```python
from build123d import *

# Parameters (mm, degrees)
BOSS_EXTRUDE4_DEPTH  = 1.5875
M3_CLEARANCE_HOLE3_D = 3
M3_CLEARANCE_HOLE1_D = 3.1
M3_CLEARANCE_HOLE4_D = 2.95
M3_CLEARANCE_HOLE2_D = 3.1
BOSS_EXTRUDE6_DEPTH  = 3.175
FILLET1_R            = 2
FILLET3_R            = 1
FILLET6_R            = 0.5
SKETCH28_W           = 54.5
SKETCH28_H           = 45
CUT_EXTRUDE4_DEPTH   = 10
CUT_EXTRUDE5_DEPTH   = 10
SKETCH30_W           = 42
SKETCH30_H           = 26
CUT_EXTRUDE6_DEPTH   = 10
SKETCH31_R           = 1.5
CUT_EXTRUDE7_DEPTH   = 10
SKETCH34_R           = 1
CUT_EXTRUDE9_DEPTH   = 10
SKETCH35_R           = 1.5
CUT_EXTRUDE10_DEPTH  = 121.250075508


with BuildPart() as part:
    # Sketch1 → Boss-Extrude4 (new, symmetric)
    with BuildSketch(Plane(origin=(0, 0, 0), x_dir=(1, 0, 0), z_dir=(0, 1, 0))):
        with BuildLine():
            Line((-62.799553621, 32.496136604), (-73.969425011, 32.691107434))
            Line((-73.969425011, 32.691107434), (-77.053684287, 35.88495141))
            ThreePointArc((-77.053684287, 35.88495141), (-84.36642289, 10.358894189), (-83.446216027, -16.178041625))
            Line((-83.446216027, -16.178041625), (-79.680911643, -13.825218315))
            Line((-79.680911643, -13.825218315), (-69.484649137, -16.179210996))
            Line((-69.484649137, -16.179210996), (-43.894490772, -57.132025032))
            Line((-43.894490772, -57.132025032), (-43.894490772, -64.826600275))
            Line((-43.894490772, -64.826600275), (-43.094490772, -64.826600275))
            Line((-43.094490772, -64.826600275), (-34, -64.826600275))
            Line((-34, -64.826600275), (-34, -62.55))
            Line((-34, -62.55), (-34, -61.55))
            Line((-34, -61.55), (-20, -61.55))
            Line((-20, -61.55), (-19.859459165, -62.55))
            Line((-19.859459165, -62.55), (19.859459165, -62.55))
            Line((19.859459165, -62.55), (20, -61.55))
            Line((20, -61.55), (34, -61.55))
            Line((34, -61.55), (34, -62.55))
            Line((34, -62.55), (34, -64.826600275))
            Line((34, -64.826600275), (43.094490772, -64.826600275))
            Line((43.094490772, -64.826600275), (43.894490772, -64.826600275))
            Line((43.894490772, -64.826600275), (43.894490772, -57.132025032))
            Line((43.894490772, -57.132025032), (69.484649137, -16.179210996))
            Line((69.484649137, -16.179210996), (79.680911643, -13.825218315))
            Line((79.680911643, -13.825218315), (83.446216027, -16.178041625))
            ThreePointArc((83.446216027, -16.178041625), (84.610662337, -8.126242604), (85, 0))
            ThreePointArc((85, 0), (82.98964744, 18.377116688), (77.053684287, 35.88495141))
            Line((77.053684287, 35.88495141), (73.969425011, 32.691107434))
            Line((73.969425011, 32.691107434), (62.799553621, 32.496136604))
            Line((62.799553621, 32.496136604), (30.284668021, 63.895396642))
            Line((30.284668021, 63.895396642), (30.089697191, 75.065268032))
            Line((30.089697191, 75.065268032), (33.173956467, 78.259112008))
            ThreePointArc((33.173956467, 78.259112008), (0, 85), (-33.173956467, 78.259112008))
            Line((-33.173956467, 78.259112008), (-30.089697191, 75.065268032))
            Line((-30.089697191, 75.065268032), (-30.284668021, 63.895396642))
            Line((-30.284668021, 63.895396642), (-62.799553621, 32.496136604))
        make_face()
    extrude(amount=BOSS_EXTRUDE4_DEPTH, both=True)

    # M3 Clearance Hole3 (through all)
    with Locations(Plane(origin=(0, -1.5875, 0), x_dir=(-1, 0, 0), z_dir=(0, -1, 0))):
        with Locations((36.5, -50), (36.5, -38), (-36.5, -50), (-36.5, -38)):
            Hole(M3_CLEARANCE_HOLE3_D / 2)

    # M3 Clearance Hole1 (through all)
    with Locations(Plane(origin=(0, 1.5875, 0), x_dir=(1, 0, 0), z_dir=(0, 1, 0))):
        with Locations((-78.542321426, -8.49139241), (78.542321426, -8.49139241), (74.155025063, 27.240269049), (-74.155025063, 27.240269049)):
            Hole(M3_CLEARANCE_HOLE1_D / 2)

    # M3 Clearance Hole4 (through all)
    with Locations(Plane(origin=(0, -1.5875, 0), x_dir=(-1, 0, 0), z_dir=(0, -1, 0))):
        with Locations((-67.099301622, -15.278865202), (-50.141885166, -42.416404279), (-61.062544382, 30.698137949), (-38.043670771, 52.927205804), (50.141885166, -42.416404279), (67.099301622, -15.278865202), (38.043670771, 52.927205804), (61.062544382, 30.698137949)):
            Hole(M3_CLEARANCE_HOLE4_D / 2)

    # M3 Clearance Hole2 (through all)
    with Locations(Plane(origin=(0, 1.5875, 0), x_dir=(1, 0, 0), z_dir=(0, 1, 0))):
        with Locations((27, 76.497766718), (-27, 76.497766718)):
            Hole(M3_CLEARANCE_HOLE2_D / 2)

    # Sketch22 → Boss-Extrude6 (add)
    with BuildSketch(Plane(origin=(0, 1.5875, 0), x_dir=(1, 0, 0), z_dir=(0, 1, 0))):
        Polygon((65.061950694, 32.535626892), (30.245177733, 66.157793715), (30.284668021, 63.895396642), (62.799553621, 32.496136604), align=None)
        Polygon((-30.284668021, 63.895396642), (-30.245177733, 66.157793715), (-65.061950694, 32.535626892), (-62.799553621, 32.496136604), align=None)
        Polygon((43.894490772, -60.151352895), (71.689396914, -15.670204865), (69.484649137, -16.179210996), (43.894490772, -57.132025032), align=None)
        Polygon((-69.484649137, -16.179210996), (-71.689396914, -15.670204865), (-43.894490772, -60.151352895), (-43.894490772, -57.132025032), align=None)
    extrude(amount=-BOSS_EXTRUDE6_DEPTH)

    # Fillet1
    fillet1_edges = [part.edges().sort_by_distance(p)[0] for p in [
        (-30.245177733, 0.79375, -66.157793715),
        (-65.061950694, 0.79375, -32.535626892),
        (-71.689396914, 0.79375, 15.670204865),
        (-43.894490772, 0.79375, 60.151352895),
        (43.894490772, -0.79375, 60.151352895),
        (71.689396914, -0.79375, 15.670204865),
        (65.061950694, 0.79375, -32.535626892),
        (30.245177733, -0.79375, -66.157793715),
        (30.089697191, -0.79375, -75.065268032),
        (73.969425011, -0.79375, -32.691107434),
        (79.680911643, -0.79375, 13.825218315),
        (-79.680911643, -0.79375, 13.825218315),
        (-73.969425011, -0.79375, -32.691107434),
        (-30.089697191, -0.79375, -75.065268032),
    ]]
    fillet(fillet1_edges, radius=FILLET1_R)

    # Fillet3
    fillet3_edges = [part.edges().sort_by_distance(p)[0] for p in [
        (33.173956467, -0.79375, -78.259112008),
        (77.053684287, 0.79375, -35.88495141),
        (83.446216027, -0.79375, 16.178041625),
        (43.894490772, -0.79375, 64.826600275),
        (34, 0.79375, 64.826600275),
        (34, -0.79375, 61.55),
        (-34, -0.79375, 61.55),
        (-34, 0.79375, 64.826600275),
        (-43.894490772, -0.79375, 64.826600275),
        (-83.446216027, -0.79375, 16.178041625),
        (-77.053684287, -0.79375, -35.88495141),
        (-33.173956467, -0.79375, -78.259112008),
    ]]
    fillet(fillet3_edges, radius=FILLET3_R - 0.0001)  # a hair under: the kernel refuses the full size

    # Fillet6
    fillet6_edges = [part.edges().sort_by_distance(p)[0] for p in [
        (20, -0.79375, 61.55),
        (19.859459165, -0.79375, 62.55),
        (-19.859459165, 0.79375, 62.55),
        (-20, 0.79375, 61.55),
    ]]
    fillet(fillet6_edges, radius=FILLET6_R)

    # Sketch28 → Cut-Extrude4 (cut)
    with BuildSketch(Plane(origin=(0, 1.5875, 0), x_dir=(1, 0, 0), z_dir=(0, 1, 0))):
        with Locations((0, -40.05)):
            Rectangle(SKETCH28_W, SKETCH28_H)
    extrude(amount=-CUT_EXTRUDE4_DEPTH, mode=Mode.SUBTRACT)

    # Sketch29 → Cut-Extrude5 (cut)
    with BuildSketch(Plane(origin=(0, 1.5875, 0), x_dir=(1, 0, 0), z_dir=(0, 1, 0))):
        with BuildLine():
            ThreePointArc((-31.5, -56.8), (-30, -58.3), (-28.5, -56.8))
            Line((-28.5, -56.8), (-30, -56.8))
            Line((-30, -56.8), (-31.5, -56.8))
        make_face()
        with BuildLine():
            Line((-30, -56.8), (-28.5, -56.8))
            ThreePointArc((-28.5, -56.8), (-30, -55.3), (-31.5, -56.8))
            Line((-31.5, -56.8), (-30, -56.8))
        make_face()
        with BuildLine():
            ThreePointArc((28.5, -56.8), (30, -58.3), (31.5, -56.8))
            ThreePointArc((31.5, -56.8), (30, -55.3), (28.5, -56.8))
        make_face()
    extrude(amount=-CUT_EXTRUDE5_DEPTH, mode=Mode.SUBTRACT)

    # Sketch30 → Cut-Extrude6 (cut)
    with BuildSketch(Plane(origin=(0, 1.5875, 0), x_dir=(1, 0, 0), z_dir=(0, 1, 0))):
        with Locations((0, -4.55)):
            Rectangle(SKETCH30_W, SKETCH30_H)
    extrude(amount=-CUT_EXTRUDE6_DEPTH, mode=Mode.SUBTRACT)

    # Sketch31 → Cut-Extrude7 (cut)
    with BuildSketch(Plane(origin=(0, 1.5875, 0), x_dir=(1, 0, 0), z_dir=(0, 1, 0))):
        with Locations(Location((-26, -14.8, 0), (0, 0, 270))):
            Circle(SKETCH31_R)
        with Locations(Location((26, -14.8, 0), (0, 0, 270))):
            Circle(SKETCH31_R)
    extrude(amount=-CUT_EXTRUDE7_DEPTH, mode=Mode.SUBTRACT)

    # Sketch34 → Cut-Extrude9 (cut)
    with BuildSketch(Plane(origin=(0, 1.5875, 0), x_dir=(1, 0, 0), z_dir=(0, 1, 0))):
        with Locations(Location((-12, 38.45, 0), (0, 0, 270))):
            Circle(SKETCH34_R)
        with Locations(Location((12, 38.45, 0), (0, 0, 270))):
            Circle(SKETCH34_R)
    extrude(amount=-CUT_EXTRUDE9_DEPTH, mode=Mode.SUBTRACT)

    # Sketch35 → Cut-Extrude10 (cut, through all)
    with BuildSketch(Plane(origin=(0, 1.5875, 0), x_dir=(1, 0, 0), z_dir=(0, 1, 0))):
        with Locations(Location((-23.5, 11.55, 0), (0, 0, 270))):
            Circle(SKETCH35_R)
        with Locations(Location((23.5, 11.55, 0), (0, 0, 270))):
            Circle(SKETCH35_R)
    extrude(amount=-CUT_EXTRUDE10_DEPTH, mode=Mode.SUBTRACT)


solid = part.part
```
Input: part model. Units: mm. Frame: model coordinates. Coordinates: 2 decimals unless noted, no trailing zeros. Loops run counter-clockwise (first coordinate to the right, second up) from the corner with the lowest first, then second, coordinate; pieces in that order, holes last. Notation, with made-up numbers: M -9.5,33.25 L 16.5,33.25 A7 ccw 16.5,43.25 Z; hole C -13.75,0.5 d8. An arc over 180 degrees is marked long. Answer in a Markdown table with one row per item.
1. Material intervals for line 1 (Z direction, x = 36.5, y = 0.3); line 2 (X direction, y = -0.1, z = -77.5); line 3 (Z direction, x = -1, y = -0.55), sorted ascending.
Response:
| item | result |
|---|---|
| line 1 | z = -60.12 to 36.5, 39.5 to 48.5, 51.5 to 64.83 |
| line 2 | x = -32.35 to -28.18, -25.82 to 25.82, 28.18 to 32.35 |
| line 3 | z = -84.99 to -8.45 |
2. Section A-A, the plane y = 1.05. Count the separate pieces of the cut face and the enclosed holes in it, then the cut area to 3 significant figures.
Response:
| item | result |
|---|---|
| separate pieces | 1 |
| enclosed holes | 26 |
| area | 13,900 mm2 |
3. Section B-B, the plane x = -6. Output: boundary loops of the cut face in (y, z), then the cut area to 3 significant figures.
Response:
| item | result |
|---|---|
| outline | M -1.59,-84.79 L 1.59,-84.79 L 1.59,-8.45 L -1.59,-8.45 Z |
| area | 242 mm2 |
4. First-contact query: pin 1 (4 mm diameter, centred on x = -36.5, z = 38, fed in from -Y); pin 2 (1 mm diameter, centred on x = 29, y = 0, fed in from +Z); pin 3 (1.5 mm diameter, centred on x = -62.5, y = -1, fed in from +Z). Flat tips, straight axial feed; report the tip coordinate or a pass-through.
Response:
| item | result |
|---|---|
| pin 1 | stops at y = -1.59 |
| pin 2 | stops at z = 61.55 |
| pin 3 | stops at z = 31.58 |
